from build123d import *

# Parameters (mm, degrees)
CROQUIS1_W              = 19
CROQUIS1_H              = 19
SALIENTE_EXTRUIR1_DEPTH = 4
CROQUIS2_W              = 14
CROQUIS2_H              = 14
CORTAR_EXTRUIR1_DEPTH   = 4
SALIENTE_EXTRUIR2_DEPTH = 4
CROQUIS9_W              = 6
CROQUIS9_H              = 6
SALIENTE_EXTRUIR6_DEPTH = 20
CROQUIS11_W             = 3.15
CROQUIS11_H             = 3.15
CORTAR_EXTRUIR3_DEPTH   = 20
REDONDEO1_R             = 3
REDONDEO2_R             = 3
REDONDEO3_R             = 3
REDONDEO6_R             = 1
REDONDEO7_R             = 1
SALIENTE_EXTRUIR7_START = -4
CROQUIS12_W             = 65
CROQUIS12_H             = 25
CROQUIS12_W_2           = 14
CROQUIS12_H_2           = 14
SALIENTE_EXTRUIR7_DEPTH = 4
CROQUIS13_W             = 65
CROQUIS13_H             = 25
CROQUIS13_W_2           = 60
CROQUIS13_H_2           = 22.4
SALIENTE_EXTRUIR8_DEPTH = 19.5
CROQUIS15_W             = 3.15
CROQUIS15_H             = 3.15
CORTAR_EXTRUIR4_DEPTH   = 20


with BuildPart() as part:
    # Croquis1 → Saliente-Extruir1 (new body)
    with BuildSketch(Plane(origin=(0, 0, 0), x_dir=(1, 0, 0), z_dir=(0, 1, 0))):
        Rectangle(CROQUIS1_W, CROQUIS1_H)
    extrude(amount=SALIENTE_EXTRUIR1_DEPTH)

    # Croquis2 → Cortar-Extruir1 (cut)
    with BuildSketch(Plane(origin=(0, 4, 0), x_dir=(1, 0, 0), z_dir=(0, 1, 0))):
        with Locations((-0.75, 1.5)):
            Rectangle(CROQUIS2_W, CROQUIS2_H)
    extrude(amount=-CORTAR_EXTRUIR1_DEPTH, mode=Mode.SUBTRACT)

    # Croquis3 → Saliente-Extruir2 (add)
    with BuildSketch(Plane(origin=(0, 4, 0), x_dir=(1, 0, 0), z_dir=(0, 1, 0))):
        Polygon((-9.5, 9.5), (-31.5, 5.730831712), (-31.5, 0.051028536), (-9.5, -2.5), align=None)
    extrude(amount=-SALIENTE_EXTRUIR2_DEPTH)

    # Croquis9 → Saliente-Extruir6 (add)
    with BuildSketch(Plane(origin=(-14.459222514, 25.211914346, -1.676631329), x_dir=(0.8679382707913074, 0.4955774572451805, -0.03295666800810758), z_dir=(-0.49667208306466687, 0.8660254037844359, -0.05759202986706984))):
        with Locations((-24.954381149, 2.785496138)):
            Rectangle(CROQUIS9_W, CROQUIS9_H)
    extrude(amount=-SALIENTE_EXTRUIR6_DEPTH)

    # Croquis11 → Cortar-Extruir3 (cut)
    with BuildSketch(Plane(origin=(-14.459222514, 25.211914346, -1.676631329), x_dir=(0.8679382707913073, 0.4955774572451806, -0.032956668008107474), z_dir=(-0.4966720830646669, 0.8660254037844358, -0.05759202986706968))):
        with Locations((-24.954381149, 2.785496138)):
            Rectangle(CROQUIS11_W, CROQUIS11_H)
    extrude(amount=-CORTAR_EXTRUIR3_DEPTH, mode=Mode.SUBTRACT)

    # Redondeo1
    redondeo1_edges = [part.edges().sort_by_distance(p)[0] for p in [
        (9.5, 2, -9.5),
        (9.5, 2, 9.5),
        (-9.5, 2, 9.5),
    ]]
    fillet(redondeo1_edges, radius=REDONDEO1_R)

    # Redondeo2
    redondeo2_edges = [part.edges().sort_by_distance(p)[0] for p in [
        (-9.5, 2, -9.5),
    ]]
    fillet(redondeo2_edges, radius=REDONDEO2_R)

    # Redondeo3
    redondeo3_edges = [part.edges().sort_by_distance(p)[0] for p in [
        (-9.5, 2, 2.5),
    ]]
    fillet(redondeo3_edges, radius=REDONDEO3_R)

    # Redondeo6
    redondeo6_edges = [part.edges().sort_by_distance(p)[0] for p in [
        (-24.54793036, -1.686293309, -5.686133961),
        (-30.661666234, 8.973960729, -6.395057355),
        (-30.547500987, 9.17302568, -0.395042751),
        (-24.433765113, -1.487228357, 0.313880643),
        (-33.755178919, 2.71233258, 0.03460334),
    ]]
    fillet(redondeo6_edges, radius=REDONDEO6_R)

    # Redondeo7
    redondeo7_edges = [part.edges().sort_by_distance(p)[0] for p in [
        (-33.755178919, 2.314202677, -5.952173136),
    ]]
    fillet(redondeo7_edges, radius=REDONDEO7_R)

    # Croquis12 → Saliente-Extruir7 (add)
    with BuildSketch(Plane(origin=(0, 4, 0), x_dir=(1, 0, 0), z_dir=(0, 1, 0)).offset(SALIENTE_EXTRUIR7_START)):
        with Locations((-0.65, 1.4)):
            Rectangle(CROQUIS12_W, CROQUIS12_H)
        with Locations((-0.75, 1.5)):
            Rectangle(CROQUIS12_W_2, CROQUIS12_H_2, mode=Mode.SUBTRACT)
    extrude(amount=SALIENTE_EXTRUIR7_DEPTH)

    # Croquis13 → Saliente-Extruir8 (add)
    with BuildSketch(Plane(origin=(0, 4, 0), x_dir=(1, 0, 0), z_dir=(0, 1, 0))):
        with Locations((-0.65, 1.4)):
            Rectangle(CROQUIS13_W, CROQUIS13_H)
        with Locations((-0.65, 1.4)):
            Rectangle(CROQUIS13_W_2, CROQUIS13_H_2, mode=Mode.SUBTRACT)
    extrude(amount=-SALIENTE_EXTRUIR8_DEPTH)

    # Croquis15 → Cortar-Extruir4 (cut)
    with BuildSketch(Plane(origin=(-14.459222514, 25.211914346, -1.676631329), x_dir=(0.8679382707913073, 0.4955774572451806, -0.032956668008107474), z_dir=(-0.4966720830646669, 0.8660254037844358, -0.05759202986706968))):
        with Locations((-24.954381149, 2.785496138)):
            Rectangle(CROQUIS15_W, CROQUIS15_H)
    extrude(amount=-CORTAR_EXTRUIR4_DEPTH, mode=Mode.SUBTRACT)


solid = part.part
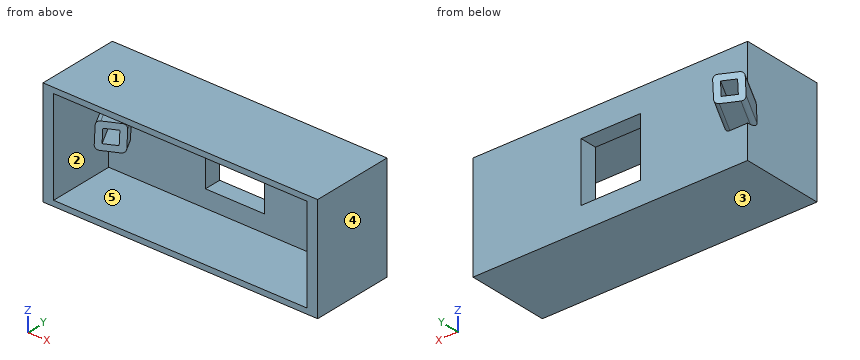
Could you check a few things on this model? Use its own coordinates, in mm. Face numbers are marked on the shaded views. A direction names the side the tool comes from. Give positions to 0.01 mm unless a question says otherwise; leave off trailing zeros. Loops run counter-clockwise (first coordinate to the right, second up) from the corner with the lowest first, then second, coordinate; pieces in that order, holes last. Notation, with made-up numbers: M 19,-28 L 75,-28 A27 ccw 75,-9 Z; hole C 77.25,17.25 d4. An arc over 180 degrees is marked long. Answer as a JSON object with one key per item and string values.
Q1. If I drill on probe 1 along Z at (x, y) = (28, -7); probe 2 along X at (y, z) = (-11.75, -1.5); probe 3 along X at (y, z) = (2.25, 5), over which ranges is the centre line in solid material (lowest first)? Write a range as [from, to].
Values found:
{"probe 1": "z = [-13.9, -12.6], [9.8, 11.1]", "probe 2": "x = [-33.15, -30.65], [29.35, 31.85]", "probe 3": "x = [-33.15, -7.75], [6.25, 31.85]"}
Q2. If we mould it in two halves opening along Z, with no side actions, what happens to the marked faces 1, 2 and 3? For each: pulls with the +Z half, pulls with the -Z half, needs draft (parallel to the pull), parting line crosses it, or undercut.
Values found:
{"face 1": "pulls with the +Z half", "face 2": "undercut", "face 3": "pulls with the -Z half"}
Q3. For P1, Ø4.5, axis at y = 2, z = -4, coming from the -X side; P2, Ø5, axis at y = -1.5, z = 0, coming from the -X side, each with a flat end and sliding along its axis, tell me the tip position at first contact or that it passes through.
Values found:
{"P1": "stops at x = -34.79", "P2": "stops at x = -33.15"}
Q4. Suppose I cut it at A-A, the plane x = -0.5. List the corners of the cut face in (y, z) for me.
Values found:
{"outline": "M -15.5,-13.9 L 4,-13.9 L 4,-8.5 L 0,-8.5 L 0,-12.6 L -15.5,-12.6 Z; M -15.5,9.8 L 0,9.8 L 0,5.5 L 4,5.5 L 4,11.1 L -15.5,11.1 Z"}
Q5. Suppose I cut it at C-C, the plane z = -10.25. List the corners of the cut face in (x, y) for me.
Values found:
{"outline": "M -33.15,-15.5 L -30.65,-15.5 L -30.65,0 L 29.35,0 L 29.35,-15.5 L 31.85,-15.5 L 31.85,4 L -33.15,4 Z"}
Q6. Suppose I cut it at B-B, the plane y = -12.25. List the corners of the cut face in (x, z) for me, plus the area to 3 significant figures.
Values found:
{"outline": "M -33.15,-13.9 L 31.85,-13.9 L 31.85,11.1 L -33.15,11.1 Z; hole M -30.65,-12.6 L 29.35,-12.6 L 29.35,9.8 L -30.65,9.8 Z", "area": "281 mm²"}
Q7. For the marked faces 4 and 5, which set-ups out of +Z, -Z, +X, -X, +Y, -Y let a thin tool reach every point of the face, with its end or its side?
Values found:
{"face 4": "+Z, -Z, +X, +Y, -Y", "face 5": "-Y"}
Q8. Suppose I cut it at D-D, the plane x = 17.5. List the corners of the cut face in (y, z) for me, plus the area to 3 significant figures.
Values found:
{"outline": "M -15.5,-13.9 L 4,-13.9 L 4,11.1 L -15.5,11.1 L -15.5,9.8 L 0,9.8 L 0,-12.6 L -15.5,-12.6 Z", "area": "140 mm²"}
